CAD build for the part. Positions are in the model's coordinates, mm. Face numbers are marked on the shaded views. A direction names the side the tool comes from. Give positions to 0.01 mm unless a question says otherwise; leave off trailing zeros. Order: outer loops, then holes, each group sorted by start corner. A loop starts at its lowest first (then second) coordinate and runs counter-clockwise, first axis right, second up. Notation, with made-up numbers: M -19.75,30.5 L 26.25,30.5 A27 cw 26.25,68.5 Z; hole C -35.5,-20.5 d9. An arc over 180 degrees is marked long. Put each result on its own line as item: value. Start each with the question number.
1) Pin check, flat tips, straight feed: pin 1 (8 mm diameter, centred on x = 3, y = -9.5, fed in from +Z); pin 2 (4 mm diameter, centred on x = 12.5, y = -8, fed in from -Z); pin 3 (10 mm diameter, centred on x = -15.5, y = 54.5, fed in from +Z). Stop position of each tip, or through.
2) Drill centre lines: line 1 (Y direction, x = 2, z = 0); line 2 (Z direction, x = 6, y = -13); line 3 (X direction, y = 17.5, z = -6.5). Where is each one in solid material? Low to high. Write a range as [from, to].
3) Cut at A-A (x = 0). Write the cut outline in (y, z), and give its area (3 significant figures).
4) Cut at B-B (x = -13.5). Write the cut outline in (y, z).
5) Tool access for the marked faces 1 and 2: list every direction of +Z, -Z, +X, -X, +Y, -Y with a clear straight run to the whole face (end or side of a thin tool).
```python
from build123d import *

# Parameters (mm, degrees)
OTW_R_12_0_12_1_D = 12
ZAOKR_GLENIE1_R   = 5
ZAOKR_GLENIE2_R   = 5
SFAZOWANIE1_SIZE  = 1


with BuildPart() as part:
    # Szkic2 → Obrót1 (revolve)
    with BuildSketch(Plane(origin=(0, 0, 0), x_dir=(1, 0, 0), z_dir=(0, 1, 0)), mode=Mode.PRIVATE) as obr_t1_sk:
        Polygon((-8, 0), (-8, 15), (-4, 15), (-4, 48.264617093), (-19.735382907, 64), (-19.735382907, 70), (-17.735382907, 70), (-15.656921938, 66.4), (-10.656921938, 66.4), (-8.578460969, 70), (-4.578460969, 70), (-2.5, 66.4), (2.5, 66.4), (4.578460969, 70), (8.578460969, 70), (10.656921938, 66.4), (15.656921938, 66.4), (17.735382907, 70), (19.735382907, 70), (19.735382907, 64), (4, 48.264617093), (4, 15), (8, 15), (8, 0), align=None)
    revolve(obr_t1_sk.sketch.rotate(Axis((-13.757967627, 0, 0), (1, 0, 0)), 180), axis=Axis((-13.757967627, 0, 0), (1, 0, 0)))  # turned: the seam where the file's is

    # Otwór Ø12.0 (12)1 (through all)
    with Locations(Plane(origin=(8, 0, 0), x_dir=(0, 0, -1), z_dir=(1, 0, 0))):
        with Locations((0, 0)):
            Hole(OTW_R_12_0_12_1_D / 2)

    # Zaokrąglenie1
    zaokr_glenie1_edges = [part.edges().sort_by_distance(p)[0] for p in [
        (4, 0, -48.264617093),
    ]]
    fillet(zaokr_glenie1_edges, radius=ZAOKR_GLENIE1_R)

    # Zaokrąglenie2
    zaokr_glenie2_edges = [part.edges().sort_by_distance(p)[0] for p in [
        (-4, 0, -48.264617093),
    ]]
    fillet(zaokr_glenie2_edges, radius=ZAOKR_GLENIE2_R)

    # Sfazowanie1
    sfazowanie1_edges = [part.edges().sort_by_distance(p)[0] for p in [
        (-8, 0, -6),
        (8, 0, -6),
    ]]
    chamfer(sfazowanie1_edges, length=SFAZOWANIE1_SIZE)


solid = part.part
```
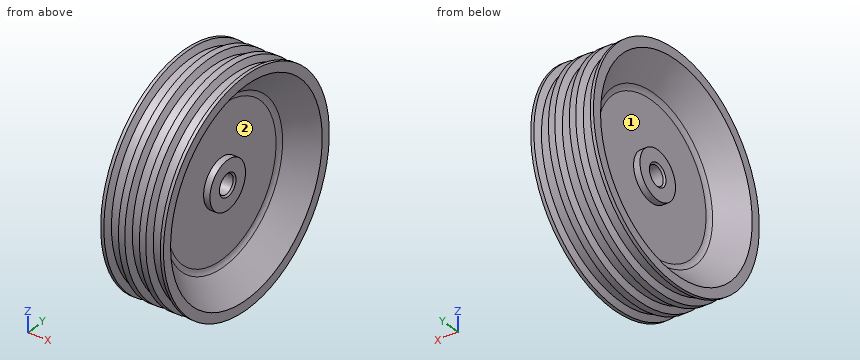
Solution:
1. pin 1: z = 69.76
1. pin 2: z = -66.2
1. pin 3: z = 48.96
2. line 1: [-66.4, -6], [6, 66.4]
2. line 2: [-68.78, -48.55], [-7.48, 7.48], [48.55, 68.78]
2. line 3: [-4, 4]
3. outline: C 0,0 d132.8; hole C 0,0 d12
3. area: 13,700 mm²
4. outline: C 0,0 d132.8; hole C 0,0 d115.53
5. face 1: -X
5. face 2: +X
